Autodesk Fusion 360 part; units mm, degrees
sketch "Name Sign LED Holder Bottom" plane through (0, 0, 0) normal (0, 1, 0) x (1, 0, 0)
  line L0 (-0.0003, -18.6907) -> (-0.0003, -13.2867)
  line L1 (32.3821, -5.4097) -> (32.3821, -0.0057)
  line L2 (-0.0003, -13.2867) -> (32.3821, -0.0057)
  line L3 (-0.0003, -18.6907) -> (32.3821, -5.4097)
  dimension "d36" = 5.404
  dimension "d37" = 5.404
  dimension "d38" = 112.3
  dimension "d39" = 35
  dimension "d40" = 4.9998
extrude "Extrude1" add sketch "Name Sign LED Holder Bottom" along normal blind 220
sketch "Magnet Holes" plane through (6.5618, 0, 15.9994) normal (0.3795, 0, 0.9252) x (0, 1, 0)
  line L0 (0, 7.0925) -> (0, -27.9075)
  line L1 (0, -27.9075) -> (220, -27.9075)
  line L2 (220, -27.9075) -> (220, 7.0925)
  line L3 (220, 7.0925) -> (0, 7.0925)
  circle A0 centre (10, -20.4075) radius 2.75
  dimension "d50" = 5.5
  dimension "d51" = 10
  dimension "d52" = 7.5
extrude "Extrude4" cut sketch "Magnet Holes" against normal blind 1.5 contours A0
pattern_linear "R-Pattern1" count 4 spacing 66.6667 along (0, 1, 0) count 2 spacing 15 along (-0.9252, 0, 0.3795) of "Extrude4"
equation "d4 = 200 mm + 10 mm + 5 mm + 5 mm"
equation "magnet_hole_diameter = 5.5 mm"
equation "magnet_hole_depth = 1.5 mm"
equation "magnet_hole_side_offset = 10 mm"
equation "magnet_hole_top_offset = 7.5 mm"
equation "magnet_pattern_length = 220.00 mm - 2 * ( magnet_hole_side_offset )"
equation "magnet_pattern_height = 35.00 mm - vertical_part_width - 2 * ( magnet_hole_top_offset )"
equation "vertical_part_width = 5.00 mm"
equation "d50 = magnet_hole_diameter"
equation "d51 = magnet_hole_side_offset"
equation "d52 = magnet_hole_top_offset"
equation "d57 = magnet_pattern_length"
equation "d58 = magnet_pattern_height"
Check sheet for the modelled part. Datum: model origin and axes. Units: mm. A direction names the side the tool comes from. Round coordinates to 2 decimals unless told otherwise and drop trailing zeros. Loops run counter-clockwise (first coordinate to the right, second up) from the corner with the lowest first, then second, coordinate; pieces in that order, holes last. Notation, with made-up numbers: (-14.75, -28) - (32.25, -28) arc R27 cw to (32.25, 3) - close; hole circle Ø3 at (82, 71). An arc over 180 degrees is marked (long way). Answer as a JSON object with one key per item and string values. Group by question number.
Q1. Sectioned sample at A-A, the plane y = 34. Enter the section's corners in (x, z).
Q2. Scan lines: line 1 along Z through (x, y) = (20, 104.5); line 2 along Z through (x, y) = (24.5, 110); line 3 along X through (y, z) = (84.5, 12.5). Record each from-to range of solid material in increasing order. Write a range as [from, to].
Q3. Sectioned sample at B-B, the plane z = 2. Enter the section's corners in (x, y), plus the area to 3 significant figures.
Q4. Set-up check for faces 4 (the face through (10.96, 76.628, 12.574)), 5 (the face through (15.96, 108.46, 6.74)): record each of +Z, -Z, +X, -X, +Y, -Y from which the full face is reachable in a straight line by a thin tool's end or side.
Q5. Gauge pin test, flat ends, axial feed: P1, Ø3, axis at y = 110, z = 16.5, coming from the +X side; P2, Ø1.5, axis at y = 154.5, z = 16.5, coming from the +X side; P3, Ø6, axis at x = 6, z = 9, coming from the +Y side; P4, Ø4, axis at x = 27.5, y = 52, coming from the +Z side. Record the tip position at first contact, or that the pin passes through.
Q6. Mould release check, pull along Z, two halves, no side actions. Record for faces 1 (the face through (10.96, 9.962, 12.574)), 2 (the face through (16, 0, 9)), 3 (the face through (15.964, 108.46, 12.143)): released by +Z, released by -Z, zero draft, split by the parting line, or undercut.
Solution:
{
 "1": {"outline": "(0, 13.29) - (32.38, 0.01) - (32.38, 5.41) - (0, 18.69) - close"},
 "2": {"line 1": "z = [5.08, 10.49]", "line 2": "z = [3.24, 8.64]", "line 3": "x = [1.92, 15.09]"},
 "3": {"outline": "(27.52, 0) - (32.38, 0) - (32.38, 220) - (27.52, 220) - close", "area": "1,070 mm²"},
 "4": {"face 4": "none", "face 5": "-Z, -X, +Y, -Y"},
 "5": {"P1": "stops at x = 9", "P2": "stops at x = 7.17", "P3": "stops at y = 220", "P4": "stops at z = 8.23"},
 "6": {"face 1": "undercut", "face 2": "zero draft", "face 3": "released by +Z"}
}
